```python
from build123d import *

# Parameters (mm, degrees)
SKETCH1_R           = 2.5
SKETCH1_R_2         = 1.5
BOSS_EXTRUDE1_DEPTH = 20
SKETCH3_R           = 2.5
CUT_EXTRUDE1_DEPTH  = 20
SKETCH4_R           = 1.5
CUT_EXTRUDE2_DEPTH  = 20


with BuildPart() as part:
    # Sketch1 → Boss-Extrude1 (new body)
    with BuildSketch(Plane.XY):
        with BuildLine():
            Line((-200.715728753, -125), (200.715728753, -125))
            ThreePointArc((200.715728753, -125), (208.3693974, -123.47759065), (214.857864376, -119.142135624))
            Line((214.857864376, -119.142135624), (243.142135624, -90.857864376))
            ThreePointArc((243.142135624, -90.857864376), (247.47759065, -84.3693974), (249, -76.715728753))
            Line((249, -76.715728753), (249, 105))
            ThreePointArc((249, 105), (243.142135624, 119.142135624), (229, 125))
            Line((229, 125), (-229, 125))
            ThreePointArc((-229, 125), (-243.142135624, 119.142135624), (-249, 105))
            Line((-249, 105), (-249, -76.715728753))
            ThreePointArc((-249, -76.715728753), (-247.47759065, -84.3693974), (-243.142135624, -90.857864376))
            Line((-243.142135624, -90.857864376), (-214.857864376, -119.142135624))
            ThreePointArc((-214.857864376, -119.142135624), (-208.3693974, -123.47759065), (-200.715728753, -125))
        make_face()
        with Locations((-199, 50)):
            Circle(SKETCH1_R, mode=Mode.SUBTRACT)
        with Locations((-102.5, 50)):
            Circle(SKETCH1_R, mode=Mode.SUBTRACT)
        with Locations(Location((102.5, 50, 0), (0, 0, 180))):
            Circle(SKETCH1_R, mode=Mode.SUBTRACT)
        with Locations(Location((199, 50, 0), (0, 0, 180))):
            Circle(SKETCH1_R, mode=Mode.SUBTRACT)
        with Locations((-9.5, 50)):
            Circle(SKETCH1_R_2, mode=Mode.SUBTRACT)
        with Locations(Location((9.5, 50, 0), (0, 0, 180))):
            Circle(SKETCH1_R_2, mode=Mode.SUBTRACT)
        with BuildLine():
            Line((116.131800265, 102.563522474), (-116.131800265, 102.563522474))
            ThreePointArc((-116.131800265, 102.563522474), (-123.202868077, 99.634590285), (-126.131800265, 92.563522474))
            Line((-126.131800265, 92.563522474), (-126.131800265, 82.389498448))
            ThreePointArc((-126.131800265, 82.389498448), (-123.202868077, 75.318430636), (-116.131800265, 72.389498448))
            Line((-116.131800265, 72.389498448), (116.131800265, 72.389498448))
            ThreePointArc((116.131800265, 72.389498448), (123.202868077, 75.318430636), (126.131800265, 82.389498448))
            Line((126.131800265, 82.389498448), (126.131800265, 92.563522474))
            ThreePointArc((126.131800265, 92.563522474), (123.202868077, 99.634590285), (116.131800265, 102.563522474))
        make_face(mode=Mode.SUBTRACT)
        with BuildLine():
            Line((-216.653872342, 102.563522474), (-167.698471554, 102.563522474))
            ThreePointArc((-167.698471554, 102.563522474), (-160.627403742, 99.634590285), (-157.698471554, 92.563522474))
            Line((-157.698471554, 92.563522474), (-157.698471554, 82.389498448))
            ThreePointArc((-157.698471554, 82.389498448), (-160.627403742, 75.318430636), (-167.698471554, 72.389498448))
            Line((-167.698471554, 72.389498448), (-216.653872342, 72.389498448))
            ThreePointArc((-216.653872342, 72.389498448), (-223.033485264, 87.476510461), (-216.653872342, 102.563522474))
        make_face(mode=Mode.SUBTRACT)
        with BuildLine():
            Line((166.318803771, 20), (-166.318803771, 20))
            ThreePointArc((-166.318803771, 20), (-171.913744739, 18.288343355), (-175.593362129, 13.739327113))
            Line((-175.593362129, 13.739327113), (-205.413984615, -60.224007784))
            ThreePointArc((-205.413984615, -60.224007784), (-205.421516172, -67.683927162), (-200.263522564, -73.073320059))
            Line((-200.263522564, -73.073320059), (-142.749435826, -99.109985162))
            ThreePointArc((-142.749435826, -99.109985162), (-140.734859414, -99.774964236), (-138.625339518, -100))
            Line((-138.625339518, -100), (138.625339518, -100))
            ThreePointArc((138.625339518, -100), (140.734859414, -99.774964236), (142.749435826, -99.109985162))
            Line((142.749435826, -99.109985162), (200.263522564, -73.073320059))
            ThreePointArc((200.263522564, -73.073320059), (205.421516172, -67.683927162), (205.413984615, -60.224007784))
            Line((205.413984615, -60.224007784), (175.593362129, 13.739327113))
            ThreePointArc((175.593362129, 13.739327113), (171.913744739, 18.288343355), (166.318803771, 20))
        make_face(mode=Mode.SUBTRACT)
        with BuildLine():
            Line((-231, 15), (-231, -24.756893222))
            ThreePointArc((-231, -24.756893222), (-227.392475088, -29.55908159), (-221.775594749, -27.431664291))
            Line((-221.775594749, -27.431664291), (-196.602681295, 12.325228931))
            ThreePointArc((-196.602681295, 12.325228931), (-196.446798009, 17.411031382), (-200.827086546, 20))
            Line((-200.827086546, 20), (-226, 20))
            ThreePointArc((-226, 20), (-229.535533906, 18.535533906), (-231, 15))
        make_face(mode=Mode.SUBTRACT)
        with BuildLine():
            Line((221.775594749, -27.431664291), (196.602681295, 12.325228931))
            ThreePointArc((196.602681295, 12.325228931), (196.446798009, 17.411031382), (200.827086546, 20))
            Line((200.827086546, 20), (226, 20))
            ThreePointArc((226, 20), (229.535533906, 18.535533906), (231, 15))
            Line((231, 15), (231, -24.756893222))
            ThreePointArc((231, -24.756893222), (227.392475088, -29.55908159), (221.775594749, -27.431664291))
        make_face(mode=Mode.SUBTRACT)
        with BuildLine():
            Line((157.698471554, 92.563522474), (157.698471554, 82.389498448))
            ThreePointArc((157.698471554, 82.389498448), (160.627403742, 75.318430636), (167.698471554, 72.389498448))
            Line((167.698471554, 72.389498448), (216.653872342, 72.389498448))
            ThreePointArc((216.653872342, 72.389498448), (223.033485264, 87.476510461), (216.653872342, 102.563522474))
            Line((216.653872342, 102.563522474), (167.698471554, 102.563522474))
            ThreePointArc((167.698471554, 102.563522474), (160.627403742, 99.634590285), (157.698471554, 92.563522474))
        make_face(mode=Mode.SUBTRACT)
    extrude(amount=BOSS_EXTRUDE1_DEPTH)

    # Sketch3 → Cut-Extrude1 (cut)
    with BuildSketch(Plane.XY.offset(20)):
        with Locations((-100, -115)):
            Circle(SKETCH3_R)
        with Locations((-120, -115)):
            Circle(SKETCH3_R)
        with Locations(Location((100, -115, 0), (0, 0, 180))):
            Circle(SKETCH3_R)
        with Locations(Location((120, -115, 0), (0, 0, 180))):
            Circle(SKETCH3_R)
    extrude(amount=-CUT_EXTRUDE1_DEPTH, mode=Mode.SUBTRACT)

    # Sketch4 → Cut-Extrude2 (cut)
    with BuildSketch(Plane.XY.offset(20)):
        with Locations((236.706992308, -60.224007784)):
            Circle(SKETCH4_R)
        with Locations((217.706992308, -60.224007784)):
            Circle(SKETCH4_R)
    extrude(amount=-CUT_EXTRUDE2_DEPTH, mode=Mode.SUBTRACT)


solid = part.part
```
Work out the finished part from the listing and answer in its coordinate system (mm). Give positions to 0.01 mm unless a question says otherwise; leave off trailing zeros. Order: outer loops, then holes, each group sorted by start corner. A loop starts at its lowest first (then second) coordinate and runs counter-clockwise, first axis right, second up. Notation, with made-up numbers: (13, 55) - (58, 55) arc R17 ccw to (58, 74) - close; hole circle Ø5 at (75.5, -1.75). An arc over 180 degrees is marked (long way). One line per item, written item: value. Start each with the question number.
1. Section B-B, the plane y = -5.5 is taken. Write down the section's boundary in (x, z).
2. For a pull along X with two mould halves and no side action, classify faces 1 (the face through (249, 13, 10)), 2 (the face through (-249, 15, 10)), 3 (the face through (223.032, 87.241, 9.86)), 4 (the face through (-2, 72.389, 10)) as released by +X, released by -X, zero draft, split by the parting line, or undercut.
3. Consider line 1 (Y direction, x = 42, z = 8.5); line 2 (Y direction, x = -220.5, z = 5.5); line 3 (Y direction, x = -199, z = 13.5). Determine where each line is inside the solid, lowest interval first.
4. Section A-A, the plane x = -69.5 is taken. Write down the section's boundary in (y, z), then the cut area to 3 significant figures.
5. Each of these flat-tipped pins is pushed along its axis until it touches: pin 1 Ø6 at (x, z) = (212, 11.5) entering from -Y; pin 2 Ø6 at (x, z) = (-212.5, 10.5) entering from -Y. Where does it stop, or does it pass through?
6. Section C-C, the plane y = -49.5 is taken. Write down the section's boundary in (x, z), then the cut area to 3 significant figures.
7. Section D-D, the plane x = 150 is taken. Write down the section's boundary in (y, z), then the cut area to 3 significant figures.
Filled sheet:
1. outline: (-249, 0) - (-231, 0) - (-231, 20) - (-249, 20) - close; (-207.89, 0) - (-183.35, 0) - (-183.35, 20) - (-207.89, 20) - close; (183.35, 0) - (207.89, 0) - (207.89, 20) - (183.35, 20) - close; (231, 0) - (249, 0) - (249, 20) - (231, 20) - close
2. face 1: released by +X
2. face 2: released by -X
2. face 3: undercut
2. face 4: undercut
3. line 1: -125 to -100, 20 to 72.39, 102.56 to 125
3. line 2: -113.5 to -25.42, 20 to 77.47, 97.48 to 125
3. line 3: -125 to -73.65, -44.32 to 8.54, 19.65 to 47.5, 52.5 to 72.39, 102.56 to 125
4. outline: (-125, 0) - (-100, 0) - (-100, 20) - (-125, 20) - close; (20, 0) - (72.39, 0) - (72.39, 20) - (20, 20) - close; (102.56, 0) - (125, 0) - (125, 20) - (102.56, 20) - close
4. area: 2,000 mm²
5. pin 1: y = -123.2
5. pin 2: y = -122.97
6. outline: (-249, 0) - (-201.09, 0) - (-201.09, 20) - (-249, 20) - close; (201.09, 0) - (249, 0) - (249, 20) - (201.09, 20) - close
6. area: 1,920 mm²
7. outline: (-125, 0) - (-95.83, 0) - (-95.83, 20) - (-125, 20) - close; (20, 0) - (125, 0) - (125, 20) - (20, 20) - close
7. area: 2,680 mm²
